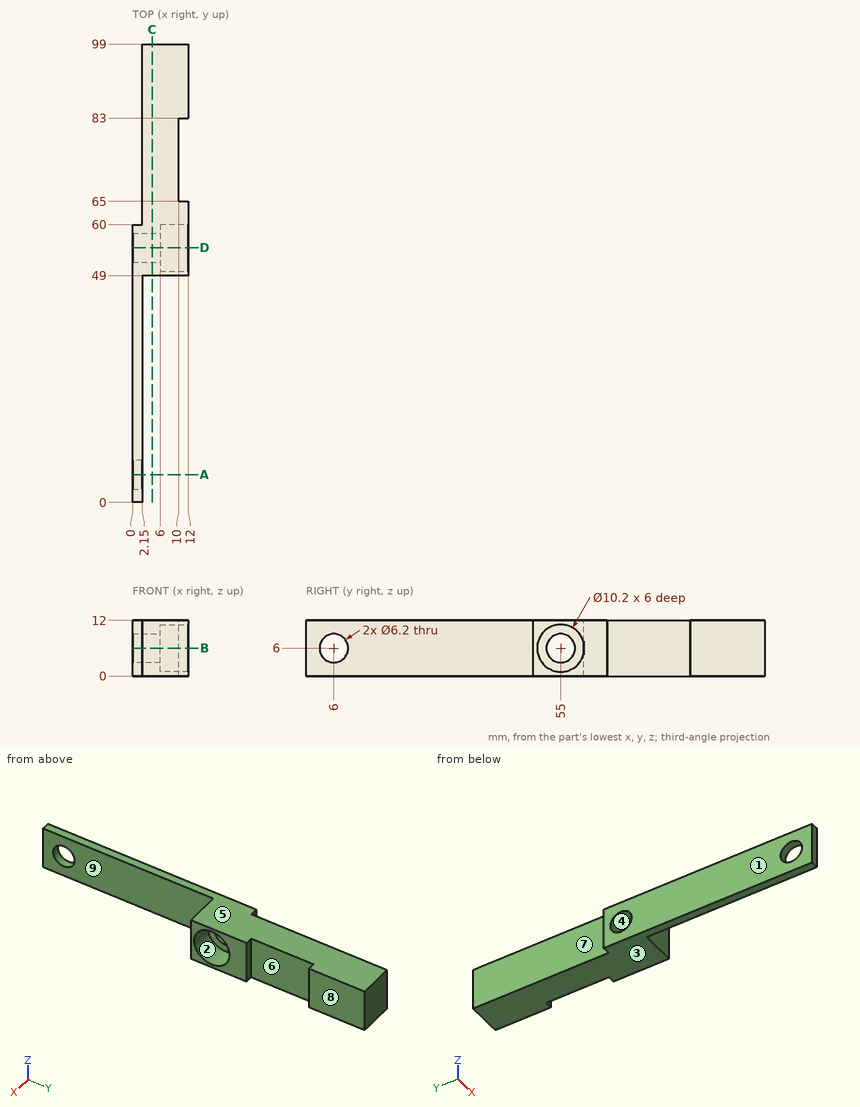
Can you work these out from the drawing? Everything is in mm from the part's minimum corner. A direction names the side the tool comes from. Coordinates: 2 decimals unless noted, no trailing zeros. Order: outer loops, then holes, each group sorted by start corner. A loop starts at its lowest first (then second) coordinate and runs counter-clockwise, first axis right, second up. Notation, with made-up numbers: (-22.75, -24) -> (28.25, -24) arc R9 ccw to (28.25, -10) -> close; hole circle Ø1 at (62, 30). An arc over 180 degrees is marked (long way). Return JSON: item names as keys, results as strings.
1) If I drill on probe 1 along Y at (x, z) = (10.75, 6.25); probe 2 along Y at (x, z) = (2.5, 6); probe 3 along Y at (x, z) = (10.75, 9.5), over which ranges is the centre line in solid material (lowest first)?
Conclusion:
{"probe 1": "y = 49 to 49.91, 60.09 to 65, 83 to 99", "probe 2": "y = 49 to 51.9, 58.1 to 99", "probe 3": "y = 49 to 51.29, 58.71 to 65, 83 to 99"}
2) I'm going to push flat-ended pins straight in: P1, Ø3, axis at x = 4, z = 5, coming from the -Y side; P2, Ø3.5, axis at y = 34.5, z = 7, coming from the +X side; P3, Ø3.5, axis at y = 75, z = 4.5, coming from the +X side. Where does each tip first touch, or does it pass through?
Conclusion:
{"P1": "stops at y = 49", "P2": "stops at x = 2.15", "P3": "stops at x = 10"}
3) If we section it at B-B on z = 6: List the corners of the cut face in (x, y) for me, plus the area to 3 significant figures.
Conclusion:
{"outline": "(0, 0) -> (2.15, 0) -> (2.15, 2.9) -> (0, 2.9) -> close; (0, 9.1) -> (2.15, 9.1) -> (2.15, 49) -> (12, 49) -> (12, 49.9) -> (6, 49.9) -> (6, 51.9) -> (0, 51.9) -> close; (0, 58.1) -> (6, 58.1) -> (6, 60.1) -> (12, 60.1) -> (12, 65) -> (10, 65) -> (10, 83) -> (12, 83) -> (12, 99) -> (2.15, 99) -> (2.15, 60) -> (0, 60) -> close", "area": "474 mm²"}
4) Thinking about a two-plate mould opening in Z: for the marked faces 1, 2, 3 and 4, which applies, +Z half, -Z half, draft (parallel to the pull), parting line (faces both ways), or undercut?
Conclusion:
{"face 1": "draft", "face 2": "undercut", "face 3": "-Z half", "face 4": "undercut"}
5) On a 3-axis mill with a long thin cutter (end or side, diameter ignored), from which of +Z, -Z, +X, -X, +Y, -Y can I reach the whole of each face in a straight line? I mean the marked faces 5, 6, 7, 8 and 9. Say none if no direction works.
Conclusion:
{"face 5": "+Z, +X, -X, +Y, -Y", "face 6": "+Z, -Z, +X", "face 7": "+Z, -Z, -X, +Y", "face 8": "+Z, -Z, +X, +Y, -Y", "face 9": "+Z, -Z, +X, -Y"}
6) If we section it at A-A on y = 6: List the corners of the cut face in (x, z) for me, plus the area to 3 significant figures.
Conclusion:
{"outline": "(0, 0) -> (2.15, 0) -> (2.15, 2.9) -> (0, 2.9) -> close; (0, 9.1) -> (2.15, 9.1) -> (2.15, 12) -> (0, 12) -> close", "area": "12.5 mm²"}
7) If we section it at C-C on x = 4.25: List the corners of the cut face in (y, z) for me.
Conclusion:
{"outline": "(49, 0) -> (99, 0) -> (99, 12) -> (49, 12) -> close; hole circle Ø6.2 at (55, 6)"}
8) If we section it at D-D on y = 55: List the corners of the cut face in (x, z) for me.
Conclusion:
{"outline": "(0, 0) -> (12, 0) -> (12, 0.9) -> (6, 0.9) -> (6, 2.9) -> (0, 2.9) -> close; (0, 9.1) -> (6, 9.1) -> (6, 11.1) -> (12, 11.1) -> (12, 12) -> (0, 12) -> close"}
